```python
from build123d import *

# Parameters (mm, degrees)
F1_DEPTH      = 2250
F3_R          = 5.4
F4_DEPTH      = 33.001
F4_DEPTH_BACK = 33.001
F6_DEPTH      = 33.001
F6_DEPTH_BACK = 33.001
F7_R          = 3.4


with BuildPart() as f1:
    # F0 (on Front) → F1 (new body, symmetric)
    with BuildSketch(Plane.XZ):
        Polygon((33, 70), (-33, 70), (-33, 61.4), (-2.85, 61.4), (-2.85, -61.4), (-33, -61.4), (-33, -70), (33, -70), (33, -61.4), (2.85, -61.4), (2.85, 61.4), (33, 61.4), align=None)
    extrude(amount=F1_DEPTH, both=True)

    # F3
    f3_edges = [f1.edges().sort_by_distance(p)[0] for p in [
        (2.85, 0, 61.4),
        (-2.85, 0, 61.4),
        (-2.85, 0, -61.4),
        (2.85, 0, -61.4),
    ]]
    fillet(f3_edges, radius=F3_R)

    # F2 (on Right) → F4 (cut, two sides)
    with BuildSketch(Plane.YZ) as f4_sk:
        Polygon((2250, 70), (450.7170761245, -1681.8248605672), (2250, -1681.8248605672), align=None)
        Polygon((450.7170761245, -1681.8248605672), (-1254.9014796783, 70), (-2250, 70), (-2250, -1681.8248605672), align=None)
    extrude(amount=-F4_DEPTH, mode=Mode.SUBTRACT)
    extrude(f4_sk.sketch, amount=F4_DEPTH_BACK, mode=Mode.SUBTRACT)

    # F5 (on Right) → F6 (cut, two sides)
    with BuildSketch(Plane.YZ) as f6_sk:
        Polygon((1738.922081788, -70), (1602.614735553, 70), (-1254.9014796783, 70), (-1118.5941334433, -70), align=None)
        Polygon((1853.8384793795, 70), (1990.1458256145, -70), (2106.2073098671, -70), (2250, 70), align=None)
    extrude(amount=-F6_DEPTH, mode=Mode.SUBTRACT)
    extrude(f6_sk.sketch, amount=F6_DEPTH_BACK, mode=Mode.SUBTRACT)

    # F7
    f7_edges = [f1.edges().sort_by_distance(p)[0] for p in [
        (-33, 1856.160788, -61.4),
        (-33, 1736.599773, 61.4),
        (33, 1856.160788, -61.4),
        (33, 1736.599773, 61.4),
    ]]
    fillet(f7_edges, radius=F7_R)


solid = f1.part
```
Check sheet for the modelled part. Datum: model origin and axes. Units: mm. A direction names the side the tool comes from. Coordinates: 2 decimals unless noted, no trailing zeros. Loops run counter-clockwise (first coordinate to the right, second up) from the corner with the lowest first, then second, coordinate; pieces in that order, holes last.
1) Sectioned sample at A-A (x = 22). Record the boundary of the cut face in (y, z), and give its area (3 significant figures).
2) Release check for a two-part mould opening along Z. For faces 4 (the face through (2.29, 1671.09, -0.33)), 5 (the face through (-19, 1854, -61.4)), 6 (the face through (0, 1726, 70)) record: released by +Z, released by -Z, zero draft, split by the parting line, or undercut.
3) Sectioned sample at B-B (y = 1800.5). Record the boundary of the cut face in (x, z).
4) Access from +Z, -Z, +X, -X, +Y, -Y to the whole of each face (thin tool, end or side, straight path). Record for faces 1 (the face through (2.85, 1794, -1)), 2 (the face through (2.3, 1921.7, 0.3)), 3 (the face through (-19, 1735, 61.4)).
5) Gauge pin test, flat ends, axial feed: pin 1 (6.5 mm diameter, centred on x = -19.5, y = 1899, fed in from +Z); pin 2 (5 mm diameter, centred on x = 9.5, y = 1921, fed in from +Z); pin 3 (12 mm diameter, centred on x = -5, z = 30, fed in from +Y); pin 4 (8 mm diameter, centred on x = -10, z = -24.5, fed in from +Y). Record the tip position at first contact, or that the pin passes through.
6) Material ranges on probe 1 along Z at (x, y) = (25.5, 1808); probe 2 along Z at (x, y) = (11, 1682); probe 3 along X at (y, z) = (1683, 1), recorded low to high.
7) Sectioned sample at D-D (z = 26). Record the boundary of the cut face in (x, y), and give its area (3 significant figures).
8) Sectioned sample at C-C (y = 1950). Record the boundary of the cut face in (x, z).
Check sheet entries:
1. outline: (1602.61, 70) - (1610.99, 61.4) - (1862.21, 61.4) - (1853.84, 70) - close; (1730.55, -61.4) - (1738.92, -70) - (1990.15, -70) - (1981.77, -61.4) - close
1. area: 4,320 mm2
2. face 4: released by -Z
2. face 5: undercut
2. face 6: released by +Z
3. outline: (-33, -70) - (33, -70) - (33, -64.8) arc R3.4 ccw to (29.6, -61.4) - (8.25, -61.4) arc R5.4 cw to (2.85, -56) - (2.85, 56) arc R5.4 cw to (8.25, 61.4) - (29.6, 61.4) arc R3.4 ccw to (33, 64.8) - (33, 70) - (-33, 70) - (-33, 64.8) arc R3.4 ccw to (-29.6, 61.4) - (-8.25, 61.4) arc R5.4 cw to (-2.85, 56) - (-2.85, -56) arc R5.4 cw to (-8.25, -61.4) - (-29.6, -61.4) arc R3.4 ccw to (-33, -64.8) - close
4. face 1: +X, +Y, -Y
4. face 2: +Z, +X, -X, +Y
4. face 3: -X, +Y, -Y
5. pin 1: stops at z = -61.4
5. pin 2: stops at z = -61.25
5. pin 3: stops at y = 1898.24
5. pin 4: passes through
6. probe 1: z = -70 to -61.4, 61.4 to 70
6. probe 2: z = 61.4 to 70
6. probe 3: x = -2.85 to 2.85
7. outline: (-2.85, 1645.45) - (2.85, 1645.45) - (2.85, 1896.68) - (-2.85, 1896.68) - close
7. area: 1,430 mm2
8. outline: (-33, -70) - (33, -70) - (33, -64.8) arc R3.4 ccw to (29.6, -61.4) - (8.25, -61.4) arc R5.4 cw to (2.85, -56) - (2.85, -28.77) - (-2.85, -28.77) - (-2.85, -56) arc R5.4 cw to (-8.25, -61.4) - (-29.6, -61.4) arc R3.4 ccw to (-33, -64.8) - close
